Design review of the part built by this model. Coordinates are the model's own, in mm. Give positions to 0.01 mm unless a question says otherwise; leave off trailing zeros. Write each loop counter-clockwise with the first axis right and the second up, starting at its lowest first coordinate (ties: lowest second). Pieces come first, ordered by that corner, then holes. Notation, with made-up numbers: (-27, 10) - (4, 10) arc R9 ccw to (4, 24) - close; hole circle Ø8 at (76.5, 9). An arc over 180 degrees is marked (long way). Write each question's results on one line, items separated by ' | '. Start each with the question number.
from build123d import *

# Parameters (mm, degrees)
BOSS_EXTRUDE1_DEPTH     = 8
BOSS_EXTRUDE2_DEPTH     = 2
SKETCH3_R               = 2.05
CUT_EXTRUDE3_DEPTH      = 10
CUT_EXTRUDE3_DEPTH_BACK = 10
FILLET2_R               = 4
SKETCH6_R               = 1.05
CUT_EXTRUDE4_DEPTH      = 3


with BuildPart() as part:
    # Sketch1 → Boss-Extrude1 (new body)
    with BuildSketch(Plane(origin=(0, 0, 0), x_dir=(1, 0, 0), z_dir=(0, 1, 0))):
        Polygon((34.518104392, -15.549979118), (32.760161227, -16.503727422), (25.996962058, -2), (22.929577374, -2), (21.996962058, 0), (27.267030045, 0), align=None)
    extrude(amount=BOSS_EXTRUDE1_DEPTH)

    # Sketch5 → Boss-Extrude2 (add)
    with BuildSketch(Plane(origin=(22.396969556, 0, -10.443878423), x_dir=(-0.422618262, 0, -0.906307787), z_dir=(0.906307787, 0, -0.422618262))):
        with BuildLine():
            Line((-40.780850255, 18.736062391), (-36.467218683, 26.428860828))
            ThreePointArc((-36.467218683, 26.428860828), (-23.692308478, 4.771999965), (-36.205658542, -17.037035395))
            Line((-36.205658542, -17.037035395), (-40.049339329, -9.057253488))
            ThreePointArc((-40.049339329, -9.057253488), (-32.517126315, 5.047276383), (-40.780850255, 18.736062391))
        make_face()
    extrude(amount=-BOSS_EXTRUDE2_DEPTH)

    # Sketch3 → Cut-Extrude3 (cut, two sides)
    with BuildSketch(Plane(origin=(20.587699136, 0, -9.600201771), x_dir=(0.422618262, 0, 0.906307787), z_dir=(-0.906307787, 0, 0.422618262))) as cut_extrude3_sk:
        with Locations((28.701516689, 4)):
            Circle(SKETCH3_R)
        with Locations((34.117040182, 18.317355913)):
            Circle(SKETCH3_R)
        with Locations((48.070293023, 24.611901983)):
            Circle(SKETCH3_R)
        with Locations((62.387648936, 19.19637849)):
            Circle(SKETCH3_R)
        with Locations((68.682195005, 5.243125649)):
            Circle(SKETCH3_R)
        with Locations((63.266671512, -9.074230264)):
            Circle(SKETCH3_R)
        with Locations((49.313418672, -15.368776333)):
            Circle(SKETCH3_R)
        with Locations((34.996062759, -9.953252841)):
            Circle(SKETCH3_R)
    extrude(amount=CUT_EXTRUDE3_DEPTH, mode=Mode.SUBTRACT)
    extrude(cut_extrude3_sk.sketch, amount=-CUT_EXTRUDE3_DEPTH_BACK, mode=Mode.SUBTRACT)

    # Fillet2
    fillet2_edges = [part.edges().sort_by_distance(p)[0] for p in [
        (31.687047343, 0, 11.840592477),
        (31.60186373, 8, 11.657915631),
    ]]
    fillet(fillet2_edges, radius=FILLET2_R)

    # Sketch6 → Cut-Extrude4 (cut, through all)
    with BuildSketch(Plane.XY.offset(2)):
        with Locations((24.429577374, 6)):
            Circle(SKETCH6_R)
        with Locations((24.429577374, 2)):
            Circle(SKETCH6_R)
    extrude(amount=-CUT_EXTRUDE4_DEPTH, mode=Mode.SUBTRACT)


solid = part.part
Q1. Add section A-A on x = 24. State the section outline as (y, z) points, plus the area to 3 significant figures.
Q2. Add section B-B on z = 5.5. State the section outline as (x, y) points.
Q3. Insertion check: P1, Ø2.5, axis at x = 24.43, y = 2, coming from the +Z side; P2, Ø10, axis at y = 13, z = 10, coming from the -X side; P3, Ø10, axis at x = 26, z = 4.5, coming from the +Y side; P4, Ø1.3, axis at x = 24.43, y = 6, coming from the +Z side. Each pin has a flat end and moves straight along its axis. Give the tip position at first contact, or say it passes through.
Q4. For line 1 along Z through (x, y) = (25.75, 2); line 2 along Z through (x, y) = (32.75, 3.5); line 3 along X through (y, z) = (-5, 21), list the stretches that pass through material, from the lowest coordinate up. Write a range as [from, to].
Q5. Add section D-D on y = 21. State the section outline as (x, z) points, plus the area to 3 significant figures.
Q6. The part is to be moulded in two halves that separate along Y. For faces 1 (the face through (24, 4, 2)), 2 (the face through (37.094, -9.337, 23.474)), 3 (the face through (37.605, -13.103, 24.504)), say which applies: +Y half, -Y half, draft (parallel to the pull), parting line (faces both ways), or undercut.
Result:
1) outline: (0, 0) - (1.04, 0) - (1.04, 2) - (0, 2) - close; (2.96, 0) - (5.04, 0) - (5.04, 2) - (2.96, 2) - close; (6.96, 0) - (8, 0) - (8, 2) - (6.96, 2) - close | area: 8.34 mm²
2) outline: (27.63, 0) - (29.83, 0) - (29.83, 8) - (27.63, 8) - close
3) P1: stops at z = 2 | P2: stops at x = 29.5 | P3: stops at y = 8 | P4: passes through
4) line 1: z = [0, 2] | line 2: z = [11.76, 14.2] | line 3: x = [34.85, 37.06]
5) outline: (33.18, 17.41) - (34.99, 16.57) - (39.1, 25.37) - (37.28, 26.21) - close | area: 19.4 mm²
6) face 1: draft | face 2: undercut | face 3: -Y half
